Check sheet for the modelled part. Datum: model origin and axes. Units: mm. Give positions to 0.01 mm unless a question says otherwise; leave off trailing zeros. Write each loop counter-clockwise with the first axis right and the second up, starting at its lowest first coordinate (ties: lowest second). Pieces come first, ordered by that corner, then holes. Notation, with made-up numbers: M 28.5,61.25 L 48.5,61.25 A27 cw 48.5,90.25 Z; hole C 5,13 d3. An arc over 180 degrees is marked long. Write item = value, one per line. Start each with the question number.
1) Mould release check, pull along Z, two halves, no side actions. Record for faces 1 (the cylindrical face through (-39.532, 40.124, -47.641)), 2 (the flat face through (-38.053, 26.8, -46.3)), 3 (the cylindrical face through (-39.574, 24.468, 46.737)): released by +Z, released by -Z, zero draft, split by the parting line, or undercut.
2) Cross-section at A-A, the plane y = 9.75. Record the cut outline in (x, z), plus the area to 3 significant figures.
3) Scan lines: line 1 along Y through (x, z) = (-39.5, 0); line 2 along Z through (x, y) = (-38.6, -11); line 3 along Y through (x, z) = (-38.3, 42). Record each from-to range of solid material in increasing order. Write a range as [from, to].
4) Cross-section at B-B, the plane z = -35. Record the cut outline in (x, y).
5) Cross-section at C-C, the plane x = -39.1. Record the cut outline in (y, z), plus the area to 3 significant figures.
```python
from build123d import *

# Parameters (mm, degrees)
SKIZZE1_W                        = 3
SKIZZE1_H                        = 52.95
F_4_7_4_7_DURCHMESSER_BOHRUNG1_D = 4.7
SKIZZE5_RX                       = 25
SKIZZE5_RY                       = 10
SCHNITT_LINEAR_AUSTRAGEN1_DEPTH  = 3
KREISMUSTER1_COUNT               = 4
CUT_EXTRUDE1_REACH               = 5
SKETCH1_R                        = 49


with BuildPart() as part:
    # Skizze1 → Rotation1 (revolve)
    with BuildSketch(Plane.XY):
        with Locations((-39.553372853, 39.775)):
            Rectangle(SKIZZE1_W, SKIZZE1_H)
    revolve(axis=Axis((-17.6629112, 9.75, 0), (-1, 0, 0)))

    # Ø4.7 (4.7) Durchmesser Bohrung1 (through all)
    with Locations(Plane(origin=(-41.053372853, 11.968723204, 19.868936148), x_dir=(0, 0, 1), z_dir=(-1, 0, 0))):
        with Locations((-13.504975118, -8.582684234), (-26.232897179, -8.582684234), (-26.232897179, 4.145237827), (-13.504975118, 4.145237827)):
            Hole(F_4_7_4_7_DURCHMESSER_BOHRUNG1_D / 2)

    # Skizze5 → Schnitt-Linear austragen1 (cut)
    with BuildSketch(Plane(origin=(-38.053372853, 0, 0), x_dir=(0, 0, -1), z_dir=(1, 0, 0))):
        with Locations(Location((-23.027329597, 32.684515508), (0, 0, 45.090609512))):
            Ellipse(SKIZZE5_RX, SKIZZE5_RY)
    schnitt_linear_austragen1 = extrude(amount=-SCHNITT_LINEAR_AUSTRAGEN1_DEPTH, mode=Mode.SUBTRACT)

    # Kreismuster1: Schnitt-Linear austragen1 ×4 about axis
    kreismuster1_axis = Axis((0, 9.75, 0), (-1, 0, 0))
    for i in range(1, KREISMUSTER1_COUNT):
        add(schnitt_linear_austragen1.rotate(kreismuster1_axis, i * 360 / KREISMUSTER1_COUNT), mode=Mode.SUBTRACT)

    # Sketch1 → Cut-Extrude1 (cut, up to next)
    with BuildSketch(Plane.ZY.offset(41.053372853), mode=Mode.PRIVATE) as cut_extrude1_sk1:
        with Locations((0, 9.75)):
            Circle(SKETCH1_R)
    cut_extrude1_tool1 = extrude(cut_extrude1_sk1.sketch, amount=-CUT_EXTRUDE1_REACH, mode=Mode.PRIVATE) & part.part
    add(cut_extrude1_tool1.solids().sort_by_distance((-41.053373, 9.75, 0))[0], mode=Mode.SUBTRACT)


solid = part.part
```
Reply:
q1.face_1 = split by the parting line
q1.face_2 = zero draft
q1.face_3 = undercut
q2.outline = M -41.05,-56.5 L -38.05,-56.5 L -38.05,-49 L -41.05,-49 Z; M -41.05,49 L -38.05,49 L -38.05,56.5 L -41.05,56.5 Z
q2.area = 45.0 mm2
q3.line_1 = [-46.75, -39.25], [58.75, 66.25]
q3.line_2 = [-52.55, -44.39], [44.39, 52.55]
q3.line_3 = [-28.04, -15.49], [34.99, 47.54]
q4.outline = M -41.05,-34.6 L -38.05,-34.6 L -38.05,-24.54 L -41.05,-24.54 Z; M -41.05,44.04 L -38.05,44.04 L -38.05,54.1 L -41.05,54.1 Z
q5.outline = C 9.75,0 d113; hole C 9.75,0 d98
q5.area = 2,490 mm2
